For this review, take the finished solid that the model builds, in its own axes (mm). A direction names the side the tool comes from. Coordinates: 2 decimals unless noted, no trailing zeros. Loops run counter-clockwise (first coordinate to the right, second up) from the corner with the lowest first, then second, coordinate; pieces in that order, holes last. Notation, with made-up numbers: M 80.5,72 L 134.5,72 A24 cw 134.5,101 Z; hole C -34,-28.5 d9. An arc over 180 degrees is marked long. Use one line per item in the form item = value.
Autodesk Inventor part; units mm, degrees
ref_plane "YZ Plane" through (0, 0, 0) normal (1, 0, 0) x (0, 1, 0)
ref_plane "XZ Plane" through (0, 0, 0) normal (0, 1, 0) x (-1, 0, 0)
ref_plane "XY Plane" through (0, 0, 0) normal (0, 0, 1) x (1, 0, 0)
sketch "Sketch1" plane through (0, 0, 0) normal (0, 0, 1) x (1, 0, 0)
  line L0 (0, 0) -> (0, 7)
  line L1 (0, 7) -> (10, 7)
  arc A0 (10, 7) -> (19.5394, 7) centre (14.7697, 8.5) ccw
  line L2 (19.5394, 7) -> (29.5394, 7)
  line L3 (29.5394, 7) -> (29.5394, 0)
  line L4 (29.5394, 0) -> (0, 0)
  dimension "d0" = 10
  dimension "d1" = 5
  dimension "d2" = 7
  dimension "d4" = 1.5
extrude "Extrusion1" add sketch "Sketch1" against normal blind 10
sketch "Sketch3" plane through (0, 0, -10) normal (0, 0, -1) x (-1, 0, 0)
  line L0 (0, 0) -> (0, 7)
  line L1 (0, 7) -> (-10, 7)
  arc A0 (-19.5394, 7) -> (-10, 7) centre (-14.7697, 8.5) ccw
  line L2 (-19.5394, 7) -> (-29.5394, 7)
  line L3 (-29.5394, 7) -> (-29.5394, 0)
  line L4 (-29.5394, 0) -> (0, 0)
  circle A1 centre (-14.7697, 8.5) radius 5
  circle A2 centre (-14.7697, 8.5) radius 8.5
  line L5 (-29.5394, 0) -> (0, 0)
extrude "Extrusion2" add sketch "Sketch3" along normal blind 20 contours A2 L2 A0 L1 | L1 A1 L2 A2
sketch "Sketch4" plane through (14.7697, 8.5, -30) normal (0, 0, -1) x (-1, 0, 0)
  line L0 (-14.7697, -8.5) -> (14.7697, -8.5)
  line L1 (0, -8.5) -> (3, -8.5)
  line L2 (0, -8.5) -> (-3, -8.5)
  circle A0 centre (0, 0) radius 5
  circle A1 centre (0, 0) radius 8.5
  line L3 (-3, -8.5) -> (3, -8.5)
  line L4 (3, -8.5) -> (3, 8.5)
  line L5 (3, 8.5) -> (-3, 8.5)
  line L6 (-3, 8.5) -> (-3, -8.5)
  dimension "d18" = 3
  dimension "d19" = 3
extrude "Extrusion3" add sketch "Sketch4" along normal blind 23.5 contours L6 A1 L0 | A1 L4 L0 | A1 L6 A0 L4 | L6 L5 A1 | A1 L4 A0 L6 | L6 A0 L4 | L5 L4 A1
sketch "Sketch6" plane through (11.7697, 4.5, -30) normal (-1, 0, 0) x (0, 0, 1)
  line L0 (0, 12.5) -> (-23.5, 12.5)
  line L1 (-11.75, 12.5) -> (-11.75, 4)
  line L2 (-11.75, 4) -> (-23.5, 4)
  circle A0 centre (-11.75, 4) radius 6.75
  circle A1 centre (-11.75, 4) radius 3
  circle A2 centre (-11.75, 4) radius 6
  point P0 (30, -4.5)
  dimension "d26" = 8.5
  dimension "d27" = 13.5
  dimension "d28" = 6
  dimension "d29" = 12
extrude "Extrusion4" cut sketch "Sketch6" against normal blind 1 contours A0 L2 A2 L1 | L1 A2 L2 A0
extrude "Extrusion5" cut sketch "Sketch6" against normal blind 4 contours A2 L2 A1 L1 | L1 A1 L2 A2
extrude "Extrusion6" cut sketch "Sketch6" against normal up to surface (6 mm away) contours A1 L2 L1 | L1 L2 A1
sketch "Sketch7" plane through (17.7697, 4.5, -30) normal (1, 0, 0) x (0, 0, -1)
  line L0 (11.75, 4) -> (23.5, 4)
  circle A0 centre (11.75, 4) radius 6.75
  line L1 (18.5, 4) -> (23.5, 4)
  circle A1 centre (19.2602, 8.1796) radius 2
  circle A2 centre (19.2602, 8.1796) radius 4
  point P0 (-30, -4.5)
  dimension "d40" = 4
  dimension "d41" = 2
extrude "Extrusion7" add sketch "Sketch7" along normal blind 5 contours A2 A0 A1 | A0 A1 A2
extrude "Extrusion8" cut sketch "Sketch7" against normal blind 2 contours A1 A0 | A0 A1
sketch "Sketch8" plane through (0, 7, 0) normal (0, 1, 0) x (1, 0, 0)
  line L0 (0, 0) -> (10, 0)
  line L1 (5, 0) -> (5, 10)
  line L2 (0, 10) -> (6.4031, 10)
  line L3 (19.5394, 0) -> (29.5394, 0)
  line L4 (24.5394, 0) -> (24.5394, 10)
  point P0 (24.5394, 5)
  point P1 (5, 5)
hole "Hole2" at (5, 7, -5) at (24.5394, 7, -5) direction (0, -1, 0) diameter 3.797 end through all
properties part number "frontChassis"
1. Consider section C-C on z = -41.75. Write out the cut boundary in (x, y), plus the area to 3 significant figures.
Computed values:
outline = M 11.77,0 L 17.77,0 L 17.77,5.5 L 15.77,5.5 L 15.77,2.5 L 12.77,2.5 L 12.77,1.75 L 11.77,1.75 Z; M 11.77,15.25 L 12.77,15.25 L 12.77,14.5 L 15.77,14.5 L 15.77,11.5 L 17.77,11.5 L 17.77,17 L 11.77,17 Z
area = 40.5 mm2
2. Tool access review of faces 4 (the face through (15, 9, -30)), 5 (the face through (12.263, 8.797, -48.493)), 6 (the face through (11.77, 16, -42)), 7 (the face through (27, 7, -5)), 8 (the face through (21, 9, -30)): name each direction out of +Z, -Z, +X, -X, +Y, -Y from which nothing blocks a thin tool from reaching the whole face with its end or side.
Computed values:
face_4 = +Z
face_5 = -X
face_6 = -Z, -X, +Y, -Y
face_7 = +Z, +X, -X, +Y
face_8 = +X, +Y, -Y
3. Consider section B-B on x = 19. Write out the cut boundary in (y, z).
Computed values:
outline = M 0,-10 L 1.13,-10 L 1.13,-30 L 5.83,-30 L 5.83,0 L 0,0 Z; C 12.68,-49.26 d8; M 11.17,-30 L 15.87,-30 L 15.87,-10 L 11.17,-10 Z; hole C 12.68,-49.26 d4
4. Consider section D-D on x = 7.5. Write out the cut boundary in (y, z), plus the area to 3 significant figures.
Computed values:
outline = M 0,-10 L 4.1,-10 L 4.1,-30 L 12.9,-30 L 12.9,-10 L 7,-10 L 7,0 L 0,0 Z
area = 246 mm2
5. Consider section A-A on z = -5. Write out the cut boundary in (x, y), plus the area to 3 significant figures.
Computed values:
outline = M 0,0 L 3.1,0 L 3.1,7 L 0,7 Z; M 6.9,0 L 22.64,0 L 22.64,7 L 19.54,7 A5 cw 10,7 L 6.9,7 Z; M 26.44,0 L 29.54,0 L 29.54,7 L 26.44,7 Z
area = 129 mm2
6. For pin 1 Ø4 at (y, z) = (13.5, -48) entering from +X; pin 2 Ø5.5 at (x, y) = (4, 3) entering from -Z; pin 3 Ø1.5 at (y, z) = (11.5, -18) entering from -X, all flat-tipped, find the tip position at first contact; note any pin that passes through.
Computed values:
pin_1 = 22.77
pin_2 = -10
pin_3 = 6.57
7. Draft analysis for pull direction Y (two halves, no side actions). For faces 1 (the face through (15.77, 13, -49)), 2 (the face through (15, 17, -42)), 3 (the face through (22.77, 12, -47)), state which applies: +Y half, -Y half, draft (parallel to the pull), parting line (faces both ways), or undercut.
Computed values:
face_1 = undercut
face_2 = +Y half
face_3 = draft
8. Wall thickness on line 1 along X through (y, z) = (8.75, -26.5); line 2 along X through (y, z) = (10.5, -35.5); line 3 along X through (y, z) = (10, -49): over which ranges is each line inside the solid? List them lowest first. Write a range as from..to.
Computed values:
line_1 = 6.27..9.78, 19.76..23.27
line_2 = 12.77..17.77
line_3 = 11.77..22.77
